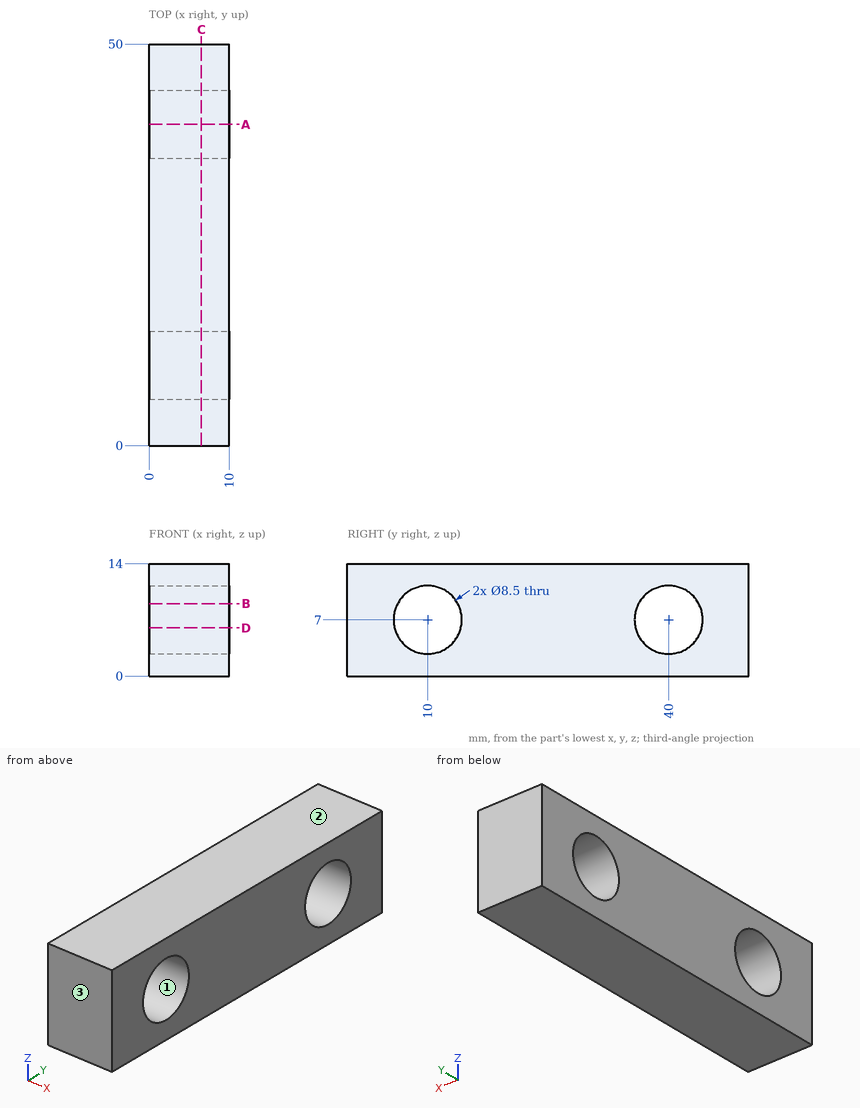
Part print with two shaded views. Sizes in mm from the minimum x, y, z corner. Coordinates: 2 decimals unless noted, no trailing zeros. Write each loop counter-clockwise with the first axis right and the second up, starting at its lowest first coordinate (ties: lowest second). Pieces come first, ordered by that corner, then holes.
(1) Cut at A-A on y = 40. List the corners of the cut face in (x, z).
(2) Pin check, flat tips, straight feed: pin 1 Ø5 at (y, z) = (19, 6.5) entering from -X; pin 2 Ø7.5 at (y, z) = (10, 7) entering from -X. Stop position of each tip, or through.
(3) Cut at C-C on x = 6.5. List the corners of the cut face in (y, z).
(4) Cut at D-D on z = 6. List the corners of the cut face in (x, y).
(5) Cut at B-B on z = 9. List the corners of the cut face in (x, y).
(6) Mould opens along Z. For the marked faces 1, 2 and 3 say: pulls with the +Z half, pulls with the -Z half, needs draft (parallel to the pull), parting line crosses it, or undercut.
(7) Drill centre lines: line 1 (Z direction, x = 2.5, y = 40); line 2 (Y direction, x = 2.5, z = 3.5); line 3 (Y direction, x = 3.25, z = 10.75). Where is each one in solid material? Low to high.
Working result:
1. outline: (0, 0) - (10, 0) - (10, 2.75) - (0, 2.75) - close; (0, 11.25) - (10, 11.25) - (10, 14) - (0, 14) - close
2. pin 1: stops at x = 0
2. pin 2: passes through
3. outline: (0, 0) - (50, 0) - (50, 14) - (0, 14) - close; hole circle Ø8.5 at (10, 7); hole circle Ø8.5 at (40, 7)
4. outline: (0, 0) - (10, 0) - (10, 5.87) - (0, 5.87) - close; (0, 14.13) - (10, 14.13) - (10, 35.87) - (0, 35.87) - close; (0, 44.13) - (10, 44.13) - (10, 50) - (0, 50) - close
5. outline: (0, 0) - (10, 0) - (10, 6.25) - (0, 6.25) - close; (0, 13.75) - (10, 13.75) - (10, 36.25) - (0, 36.25) - close; (0, 43.75) - (10, 43.75) - (10, 50) - (0, 50) - close
6. face 1: undercut
6. face 2: pulls with the +Z half
6. face 3: needs draft
7. line 1: z = 0 to 2.75, 11.25 to 14
7. line 2: y = 0 to 7.59, 12.41 to 37.59, 42.41 to 50
7. line 3: y = 0 to 8, 12 to 38, 42 to 50
